```python
from build123d import *

# Parameters (mm, degrees)
SKETCH1_W           = 235.4072
SKETCH1_H           = 159.2072
BOSS_EXTRUDE1_DEPTH = 3.4036
SKETCH2_W           = 3.4036
SKETCH2_H           = 155.8036
BOSS_EXTRUDE2_DEPTH = 152.4


with BuildPart() as part:
    # Sketch1 → Boss-Extrude1 (new body)
    with BuildSketch(Plane(origin=(0, 0, 0), x_dir=(1, 0, 0), z_dir=(0, 1, 0))):
        with Locations((117.7036, 79.6036)):
            Rectangle(SKETCH1_W, SKETCH1_H)
    extrude(amount=BOSS_EXTRUDE1_DEPTH)

    # Sketch2 → Boss-Extrude2 (add)
    with BuildSketch(Plane(origin=(0, 3.4036, 0), x_dir=(1, 0, 0), z_dir=(0, 1, 0))):
        Polygon((232.0036, 3.4036), (0, 3.4036), (0, 0), (235.4072, 0), (235.4072, 3.4036), align=None)
        with Locations((233.7054, 81.3054)):
            Rectangle(SKETCH2_W, SKETCH2_H)
    extrude(amount=BOSS_EXTRUDE2_DEPTH)


solid = part.part
```
Check sheet for the modelled part. Datum: model origin and axes. Units: mm. A direction names the side the tool comes from. Coordinates: 2 decimals unless noted, no trailing zeros. Order: outer loops, then holes, each group sorted by start corner. A loop starts at its lowest first (then second) coordinate and runs counter-clockwise, first axis right, second up. Notation, with made-up numbers: (-26.5, 1) -> (22.5, 1) arc R15 ccw to (22.5, 26) -> close; hole circle Ø10 at (-14, 24.5). An arc over 180 degrees is marked (long way). Write each question's results on one line, items separated by ' | '. Start each with the question number.
1) Section check A-A (x = 53). Enter the section's corners in (y, z).
2) Set-up check for faces 1 (the face through (116, 77, 0)), 2 (the face through (118, 79, -3.404)): record each of +Z, -Z, +X, -X, +Y, -Y from which the full face is reachable in a straight line by a thin tool's end or side.
3) Section check B-B (y = 143.5). Enter the section's corners in (x, z).
4) Depth check by flat-ended pin: pin 1 (5 mm diameter, centred on y = 16, z = -63.5, fed in from -X); pin 2 (5 mm diameter, centred on x = 205.5, z = -60.5, fed in from +Y). Enter the tip coordinate at first touch or a pass-through.
5) Material ranges on line 1 along Y through (x, z) = (148.5, -63); line 2 along Z through (x, y) = (161, 145); line 3 along X through (y, z) = (53, -142.5), recorded low to high.
Checked values:
1) outline: (0, -159.21) -> (3.4, -159.21) -> (3.4, -3.4) -> (155.8, -3.4) -> (155.8, 0) -> (0, 0) -> close
2) face 1: +Z, +X, -X, +Y, -Y | face 2: -Z, -X, +Y
3) outline: (0, -3.4) -> (232, -3.4) -> (232, -159.21) -> (235.41, -159.21) -> (235.41, 0) -> (0, 0) -> close
4) pin 1: x = 232 | pin 2: y = 3.4
5) line 1: 0 to 3.4 | line 2: -3.4 to 0 | line 3: 232 to 235.41
